Check sheet for the modelled part. Datum: model origin and axes. Units: mm. A direction names the side the tool comes from. Round coordinates to 2 decimals unless told otherwise and drop trailing zeros. Write each loop counter-clockwise with the first axis right and the second up, starting at its lowest first coordinate (ties: lowest second). Pieces come first, ordered by that corner, then holes. Notation, with made-up numbers: (-10.5, 56) -> (36.5, 56) arc R17 cw to (36.5, 77) -> close; hole circle Ø10 at (-25.5, 66.5). An arc over 180 degrees is marked (long way). Answer as a JSON object with one key per item and string values. Group by question number.
```python
from build123d import *

# Parameters (mm, degrees)
F0_W        = 5.5
F0_H        = 5
F0_W_2      = 51
F0_H_2      = 51
F1_DEPTH    = 190
F2_T1_DEPTH = 215
F2_T3_DEPTH = 212.9128784748
F4_DEPTH    = 60
F6_DEPTH    = 60


# Not quite as in the source:
# - a fillet or chamfer that OpenCascade refuses, or shapes differently, is made with other operations: its cross-section is extruded or revolved along the edge and cut away or added


with BuildPart() as f1:
    # F0 (on Top) → F1 (new body)
    with BuildSketch(Plane.XY):
        Polygon((-33.5212003861, 28.1146157656), (-28.0212003861, 28.1146157656), (-28.0212003861, 33.6146157656), (-28.0212003861, 38.6146157656), (-36.5212003861, 38.6146157656), (-36.5212003861, 28.1146157656), align=None)
        Polygon((-28.0212003861, 38.6146157656), (-28.0212003861, 33.6146157656), (-23.0212003861, 33.6146157656), (-13.0212003861, 33.6146157656), (-13.0212003861, 38.6146157656), align=None)
        with Locations((-30.7712003861, 25.6146157656)):
            Rectangle(F0_W, F0_H)
        Polygon((-33.5212003861, 23.1146157656), (-33.5212003861, 28.1146157656), (-36.5212003861, 28.1146157656), (-36.5212003861, 13.1146157656), (-33.5212003861, 13.1146157656), align=None)
        Polygon((-23.0212003861, 28.1146157656), (-28.0212003861, 28.1146157656), (-28.0212003861, 23.1146157656), (-28.0212003861, -30.3853842344), (30.4787996139, -30.3853842344), (30.4787996139, 28.1146157656), align=None)
        with Locations((-0.0212003861, 0.1146157656)):
            Rectangle(F0_W_2, F0_H_2, mode=Mode.SUBTRACT)
    extrude(amount=F1_DEPTH)

    # F2: fillet of radius 5 on 4 edges, made by hand

    # F2_s2 → F2_t1 (cut)
    with BuildSketch(Plane.XY.offset(-12.5)):
        with BuildLine():
            ThreePointArc((-31.5212003861, 38.6146157656), (-35.056734292, 37.1501496716), (-36.5212003861, 33.6146157656))
            Line((-36.5212003861, 33.6146157656), (-36.5212003861, 38.6146157656))
            Line((-36.5212003861, 38.6146157656), (-31.5212003861, 38.6146157656))
        make_face()
        with BuildLine():
            ThreePointArc((-13.0212003861, 33.6146157656), (-14.4856664802, 37.1501496716), (-18.0212003861, 38.6146157656))
            Line((-18.0212003861, 38.6146157656), (-13.0212003861, 38.6146157656))
            Line((-13.0212003861, 38.6146157656), (-13.0212003861, 33.6146157656))
        make_face()
        with BuildLine():
            ThreePointArc((-18.0212003861, 33.6146157656), (-14.4856664802, 35.0790818597), (-13.0212003861, 38.6146157656))
            Line((-13.0212003861, 38.6146157656), (-13.0212003861, 33.6146157656))
            Line((-13.0212003861, 33.6146157656), (-18.0212003861, 33.6146157656))
        make_face()
    extrude(amount=F2_T1_DEPTH, mode=Mode.SUBTRACT)

    # F2_s4 → F2_t3 (cut)
    with BuildSketch(Plane.XY.offset(-11.4564392374)):
        with BuildLine():
            ThreePointArc((-36.5212003861, 17.6971914606), (-35.7045005188, 14.9585786731), (-33.5212003861, 13.1146157656))
            Line((-33.5212003861, 13.1146157656), (-36.5212003861, 13.1146157656))
            Line((-36.5212003861, 13.1146157656), (-36.5212003861, 17.6971914606))
        make_face()
    extrude(amount=F2_T3_DEPTH, mode=Mode.SUBTRACT)

    # F3 (on face) → F4 (cut)
    with BuildSketch(Plane.YZ.offset(30.4787996139)):
        with BuildLine():
            Line((-22.5, 155), (22.5, 155))
            ThreePointArc((22.5, 155), (0, 177.5), (-22.5, 155))
        make_face()
        with BuildLine():
            ThreePointArc((-22.5, 155), (0, 132.5), (22.5, 155))
            Line((22.5, 155), (-22.5, 155))
        make_face()
        with BuildLine():
            ThreePointArc((-22.5, 35), (0, 57.5), (22.5, 35))
            Line((22.5, 35), (22.5, 155))
            ThreePointArc((22.5, 155), (0, 132.5), (-22.5, 155))
            Line((-22.5, 155), (-22.5, 35))
        make_face()
        with BuildLine():
            Line((-22.5, 35), (22.5, 35))
            ThreePointArc((22.5, 35), (0, 57.5), (-22.5, 35))
        make_face()
        with BuildLine():
            ThreePointArc((-22.5, 35), (0, 12.5), (22.5, 35))
            Line((22.5, 35), (-22.5, 35))
        make_face()
    extrude(amount=-F4_DEPTH, mode=Mode.SUBTRACT)

    # F5 (on face) → F6 (cut)
    with BuildSketch(Plane.XZ.offset(30.3853842344)):
        with BuildLine():
            Line((-22.5, 145), (22.5, 145))
            ThreePointArc((22.5, 145), (0, 167.5), (-22.5, 145))
        make_face()
        with BuildLine():
            ThreePointArc((-22.5, 145), (0, 122.5), (22.5, 145))
            Line((22.5, 145), (-22.5, 145))
        make_face()
        with BuildLine():
            Line((22.5, 45), (22.5, 145))
            ThreePointArc((22.5, 145), (0, 122.5), (-22.5, 145))
            Line((-22.5, 145), (-22.5, 45))
            ThreePointArc((-22.5, 45), (0, 67.5), (22.5, 45))
        make_face()
        with BuildLine():
            Line((-22.5, 45), (22.5, 45))
            ThreePointArc((22.5, 45), (0, 67.5), (-22.5, 45))
        make_face()
        with BuildLine():
            ThreePointArc((-22.5, 45), (0, 22.5), (22.5, 45))
            Line((22.5, 45), (-22.5, 45))
        make_face()
    extrude(amount=-F6_DEPTH, mode=Mode.SUBTRACT)


solid = f1.part
```
(1) Go/stop test with flat-tipped pins: pin 1 Ø1.5 at (y, z) = (-28, 117.5) entering from -X; pin 2 Ø12 at (y, z) = (-16, 87) entering from -X; pin 3 Ø3 at (y, z) = (17, 131.5) entering from +X; pin 4 Ø1.5 at (x, z) = (27, 125) entering from +Y. Record where each tip stops, or that it passes through.
(2) Section check A-A on y = 0. Record the cut outline in (x, z), then the cut area to 4 significant figures.
(3) Scan lines: line 1 along Y through (x, z) = (-22.5, 13.5); line 2 along X through (y, z) = (-9.5, 11.5); line 3 along Y through (x, z) = (-4, 16). Record each from-to range of solid material in increasing order.
(4) Section check C-C on x = 0. Record the cut outline in (y, z), then the cut area to 4 significant figures.
(5) Section check B-B on z = 100. State how many separate pieces and enclosed holes the cut face has, then the cut area to 3 significant figures.
(6) Release check for a two-part mould opening along Y. For faces 1 (the flat face through (30.479, -28, 94)), 2 (the cylindrical face through (28.014, 0.495, 177.495)), 3 (the cylindrical face through (-35.018, 37.189, 93.67)) record: pulls with the +Y half, pulls with the -Y half, needs draft (parallel to the pull), parting line crosses it, or undercut.
(7) Access from +Z, -Z, +X, -X, +Y, -Y to the whole of each face (thin tool, end or side, straight path). Record for faces 4 (the flat face through (-23, 25.615, 95)), 5 (the cylindrical face through (-0.495, 26.847, 22.505)), 6 (the flat face through (28, 28.115, 94)), 7 (the cylindrical face through (-26.754, 0.495, 177.495)).
Data:
{
 "1": {"pin 1": "stops at x = -28.02", "pin 2": "passes through", "pin 3": "stops at x = -33.52", "pin 4": "stops at y = 28.11"},
 "2": {"outline": "(-28.02, 0) -> (-25.52, 0) -> (-25.52, 12.5) -> (-28.02, 12.5) -> close; (-28.02, 177.5) -> (-25.52, 177.5) -> (-25.52, 190) -> (-28.02, 190) -> close; (25.48, 0) -> (30.48, 0) -> (30.48, 12.5) -> (25.48, 12.5) -> close; (25.48, 177.5) -> (30.48, 177.5) -> (30.48, 190) -> (25.48, 190) -> close", "area": "187.5 mm²"},
 "3": {"line 1": "y = -30.39 to -25.39, 25.61 to 28.11, 33.61 to 38.61", "line 2": "x = -28.02 to -25.52, 25.48 to 30.48", "line 3": "y = -30.39 to -25.39, 25.61 to 28.11"},
 "4": {"outline": "(-30.39, 0) -> (-25.39, 0) -> (-25.39, 22.5) -> (-30.39, 22.5) -> close; (-30.39, 167.5) -> (-25.39, 167.5) -> (-25.39, 190) -> (-30.39, 190) -> close; (25.61, 0) -> (28.11, 0) -> (28.11, 22.5) -> (25.61, 22.5) -> close; (25.61, 167.5) -> (28.11, 167.5) -> (28.11, 190) -> (25.61, 190) -> close", "area": "337.5 mm²"},
 "5": {"separate pieces": "4", "enclosed holes": "0", "area": "364 mm²"},
 "6": {"face 1": "needs draft", "face 2": "undercut", "face 3": "pulls with the +Y half"},
 "7": {"face 4": "+Z, -Z", "face 5": "-Y", "face 6": "+Z, -Z, +X", "face 7": "+X"}
}
